Work out the finished part from the listing and answer in its coordinate system (mm). A direction names the side the tool comes from. Give positions to 0.01 mm unless a question says otherwise; leave off trailing zeros. Loops run counter-clockwise (first coordinate to the right, second up) from the corner with the lowest first, then second, coordinate; pieces in that order, holes last. Notation, with made-up numbers: (68, 2) - (118, 2) arc R21 ccw to (118, 10) - close; hole circle Ø11 at (-5.5, -20.5). An arc over 180 degrees is marked (long way). One line per question, with ' | ' between items.
from build123d import *

# Parameters (mm, degrees)
EXTRUDE_1_DEPTH = 50
EXTRUDE_START   = -2.5
EXTRUDE_2_DEPTH = 5


# Read off the part's stored shape, not the designer's step: 凸台-拉伸2
with BuildPart() as part:
    # 草图1 → 凸台-拉伸1 (new body)
    with BuildSketch(Plane.XY.offset(-25)):
        Polygon((-40, 0), (40, 0), (40, 36), (32, 36), (32, 8), (-40, 8), align=None)
    extrude(amount=EXTRUDE_1_DEPTH)

    # 凸台-拉伸2 outline → 凸台-拉伸2 (add)
    with BuildSketch(Plane.XY.offset(EXTRUDE_START)):
        Polygon((32, 32), (8, 8), (32, 8), align=None)
    extrude(amount=EXTRUDE_2_DEPTH)


solid = part.part
1. Flat-ended cylindrical pins translate along their axes: pin 1 (15 mm diameter, centred on x = -3, z = 5.5, fed in from +Y); pin 2 (5 mm diameter, centred on y = 15, z = -16.5, fed in from -X); pin 3 (19 mm diameter, centred on x = 22, y = 16.5, fed in from -Z); pin 4 (7 mm diameter, centred on x = 25.5, y = 15, fed in from +Z). Find the tip coordinate at first contact, or state that the pin passes through.
Evaluation:
pin 1: y = 8 | pin 2: x = 32 | pin 3: z = -25 | pin 4: z = 2.5
2. Find section D-D on x = -30. Write down the section's boundary in (y, z).
Evaluation:
outline: (0, -25) - (8, -25) - (8, 25) - (0, 25) - close
3. Consider L1, parallel to Y at x = 16, z = 4; L2, parallel to Z at x = 13, y = 12; L3, parallel to X at y = 12.5, z = -18. Determine where each line is inside the solid, lowest interval first.
Evaluation:
L1: 0 to 8 | L2: -2.5 to 2.5 | L3: 32 to 40
4. Find section B-B on y = 26.5. Write down the section's boundary in (x, z).
Evaluation:
outline: (26.5, -2.5) - (32, -2.5) - (32, -25) - (40, -25) - (40, 25) - (32, 25) - (32, 2.5) - (26.5, 2.5) - close
5. Find section A-A on x = 22. Write down the section's boundary in (y, z), then the cut area to 3 significant figures.
Evaluation:
outline: (0, -25) - (8, -25) - (8, -2.5) - (22, -2.5) - (22, 2.5) - (8, 2.5) - (8, 25) - (0, 25) - close | area: 470 mm2
6. Which of the six approach directions +Z, -Z, +X, -X, +Y, -Y give full straight-line access (tool end or side, diameter ignored) to faces 1 (the flat face through (-1, 0, 0)), 2 (the flat face through (25, 15, 2.5)), 3 (the flat face through (32, 22, -6)), 4 (the flat face through (25, 15, -2.5)), 5 (the flat face through (-40, 4, 0))?
Evaluation:
face 1: +Z, -Z, +X, -X, -Y | face 2: +Z, -X, +Y | face 3: -X, +Y | face 4: -Z, -X, +Y | face 5: +Z, -Z, -X, +Y, -Y
7. Find section C-C on z = 5.5. Write down the section's boundary in (x, y), then the cut area to 3 significant figures.
Evaluation:
outline: (-40, 0) - (40, 0) - (40, 36) - (32, 36) - (32, 8) - (-40, 8) - close | area: 864 mm2
